```python
from build123d import *

# Parameters (mm, degrees)
BOSS_EXTRUDE1_DEPTH     = 130.175
CUT_EXTRUDE1_DEPTH      = 198.438033
CUT_EXTRUDE1_DEPTH_BACK = 198.438033
SKETCH2_W               = 57.15
SKETCH2_H               = 74.103907915
SKETCH3_W               = 15.875
SKETCH3_H               = 34.925
CUT_EXTRUDE2_DEPTH      = 198.438033
DRAFT1_ANGLE            = -5
CUT_EXTRUDE3_DEPTH      = 188.228236601
CUT_EXTRUDE3_DEPTH_BACK = 188.228236601
SKETCH4_R               = 2.178428953


with BuildPart() as part:
    # Sketch1 → Boss-Extrude1 (new body)
    with BuildSketch(Plane(origin=(0, 0, 0), x_dir=(0, 0, -1), z_dir=(1, 0, 0))):
        with BuildLine():
            Line((0, 0), (0, 6.35))
            ThreePointArc((0, 6.35), (7.170490025, 54.477745417), (28.059114221, 98.425))
            Line((28.059114221, 98.425), (60.067057111, 98.425))
            ThreePointArc((60.067057111, 98.425), (69.592057111, 88.9), (79.117057111, 98.425))
            Line((79.117057111, 98.425), (111.125, 98.425))
            Line((111.125, 98.425), (111.125, 0))
            Line((111.125, 0), (98.425, 0))
            Line((98.425, 0), (98.425, 6.35))
            Line((98.425, 6.35), (79.375, 6.35))
            Line((79.375, 6.35), (78.839467499, 7.9375))
            Line((78.839467499, 7.9375), (40.880795395, 7.9375))
            Line((40.880795395, 7.9375), (36.174906872, 6.35))
            Line((36.174906872, 6.35), (12.7, 6.35))
            Line((12.7, 6.35), (12.7, 0))
            Line((12.7, 0), (0, 0))
        make_face()
    extrude(amount=BOSS_EXTRUDE1_DEPTH)

    # Sketch2 → Cut-Extrude1 (cut, two sides: drawn at the far end of the back side and taken through both)
    with BuildSketch(Plane(origin=(0, 0, -111.125), x_dir=(-1, 0, 0), z_dir=(0, 0, -1)).offset(-CUT_EXTRUDE1_DEPTH_BACK)):
        with Locations((-66.675, 61.373046043)):
            Rectangle(SKETCH2_W, SKETCH2_H)
    extrude(amount=CUT_EXTRUDE1_DEPTH + CUT_EXTRUDE1_DEPTH_BACK, mode=Mode.SUBTRACT)

    # Sketch3 → Cut-Extrude2 (cut, through all)
    with BuildSketch(Plane(origin=(0, 98.425, 0), x_dir=(1, 0, 0), z_dir=(0, 1, 0))):
        with Locations((122.2375, 17.4625)):
            Rectangle(SKETCH3_W, SKETCH3_H)
    extrude(amount=-CUT_EXTRUDE2_DEPTH, mode=Mode.SUBTRACT)

    # Draft1
    draft1_faces = [part.faces().sort_by_distance(p)[0] for p in [
        (1.631962354, 49.2125, -111.125),
        (122.2375, 52.3875, -34.925),
        (130.175, 51.366021229, -73.60068913),
        (114.3, 42.899391588, -20.187689821),
        (95.25, 59.043863813, -60.63952827),
        (0, 49.133887707, -59.518940982),
        (38.1, 59.043863813, -60.63952827),
    ]]
    draft(draft1_faces, Plane(origin=(130.175, 6.35, -36.174906872), x_dir=(0, 0, -1), z_dir=(0, -1, 0)), DRAFT1_ANGLE)

    # Sketch4 → Cut-Extrude3 (cut, two sides: drawn at the far end of the back side and taken through both)
    with BuildSketch(Plane(origin=(0, 24.321092085, 0), x_dir=(1, 0, 0), z_dir=(0, 1, 0)).offset(-CUT_EXTRUDE3_DEPTH_BACK)):
        with Locations(Location((42.869708487, 60.325, 0), (0, 0, 270))):
            Circle(SKETCH4_R)
    extrude(amount=CUT_EXTRUDE3_DEPTH + CUT_EXTRUDE3_DEPTH_BACK, mode=Mode.SUBTRACT)


solid = part.part
```
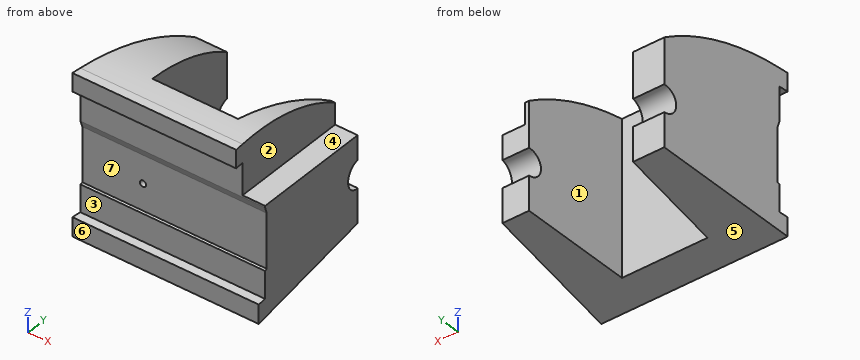
The listing builds one solid part. Answer for the finished solid, in the listing's coordinates (mm). Face numbers are marked on the shaded views. A direction names the side the tool comes from. Give positions to 0.01 mm unless a question says otherwise; leave off trailing zeros. Loops run counter-clockwise (first coordinate to the right, second up) from the corner with the lowest first, then second, coordinate; pieces in that order, holes last. Notation, with made-up numbers: (79, 83) - (122, 83) arc R29 ccw to (122, 103) - close; hole circle Ø10 at (2.5, 15). An arc over 180 degrees is marked (long way). Answer as CSV lines item,"result". Start each with the question number.
Item 1: A cutting plane is placed at A-A on y = 64. Determine the outline of the cut face in (x, z), then the cut area to 3 significant figures.
Item 2: The mould has two halves that part along Z. Classify the marked faces 4, 5, 6 and 7: +Z half, -Z half, draft (parallel to the pull), parting line (faces both ways), or undercut.
Item 3: A cutting plane is placed at B-B on z = -32. Determine the outline of the cut face in (x, y) (3 decimals).
Item 4: A cutting plane is placed at D-D on y = 92. Determine the outline of the cut face in (x, z), then the cut area to 3 significant figures.
Item 5: Each of these flat-tipped pins is pushed along its axis until it touches: pin 1 (11.5 mm diameter, centred on x = 45.5, z = -55, fed in from -Y); pin 2 (5.5 mm diameter, centred on x = 42.87, z = -60.32, fed in from +Y); pin 3 (2 mm diameter, centred on y = 14, z = -79.5, fed in from -X). Where does it stop, or does it pass through?
Item 6: For the marked faces 1, 2 and 3, determine the directions among +Z, -Z, +X, -X, +Y, -Y from which every point of the face is accessible in a straight line to the end or side of a thin tool.
Item 7: Find the intervals of material crossed by line 1 (Y direction, x = 72, z = -97); line 2 (Y direction, x = 52.5, z = -78.5); line 3 (X direction, y = 27, z = -9), in increasing order. Write a range as from..to.
Found:
1,outline,"(5.04, -106.08) - (33.06, -106.08) - (33.06, -10.39) - (5.04, -10.39) - close; (100.29, -106.08) - (125.13, -106.08) - (125.13, -39.97) - (109.26, -39.97) - (109.26, -10.39) - (100.29, -10.39) - close"
1,area,"4,590 mm^2"
2,face 4,"+Z half"
2,face 5,"-Z half"
2,face 6,"draft"
2,face 7,"undercut"
3,outline,"(0, 6.35) - (114.3, 6.35) - (106.244, 98.425) - (103.306, 98.425) - (96.822, 24.321) - (36.528, 24.321) - (30.044, 98.425) - (8.056, 98.425) - close"
4,outline,"(7.49, -103.63) - (30.61, -103.63) - (30.61, -76.62) - (7.49, -76.62) - close; (7.49, -62.56) - (30.61, -62.56) - (30.61, -23.95) - (7.49, -23.95) - close; (102.74, -103.63) - (122.68, -103.63) - (122.68, -76.62) - (102.74, -76.62) - close; (102.74, -62.56) - (122.68, -62.56) - (122.68, -42.42) - (106.81, -42.42) - (106.81, -23.95) - (102.74, -23.95) - close"
4,area,"2,530 mm^2"
5,pin 1,"stops at y = 7.94"
5,pin 2,"stops at y = 24.32"
5,pin 3,"stops at x = 0.58"
6,face 1,"+Z, -Z, +Y"
6,face 2,"+Z, +X, +Y"
6,face 3,"+X, -X, -Y"
7,line 1,"y = 6.35..24.32"
7,line 2,"y = 7.94..24.32"
7,line 3,"x = 1.81..36.29, 97.06..112.49"
